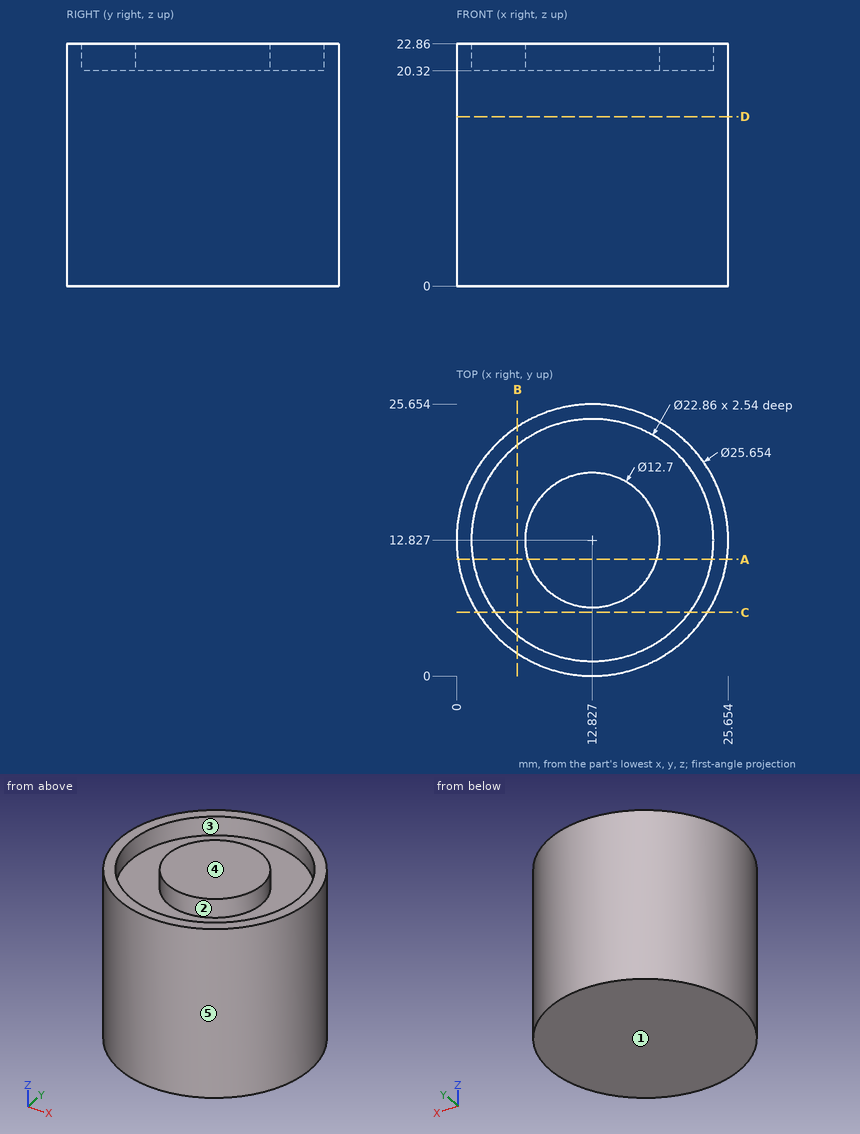
For this review, use the dimensioned drawing (mm, ordinates from the lowest corner) and the shaded views. A direction names the side the tool comes from. Coordinates: 2 decimals unless noted, no trailing zeros. Order: outer loops, then holes, each group sorted by start corner. A loop starts at its lowest first (then second) coordinate and runs counter-clockwise, first axis right, second up. Notation, with made-up numbers: M 39.25,56 L 96.25,56 A8 ccw 96.25,65 Z; hole C 85.5,78 d7. An arc over 180 degrees is marked long. Answer as a JSON object with one key per item and string values. Group by question number.
1) Add section C-C, the plane y = 6. Write out the cut boundary in (x, z).
2) Wall thickness on L1, parallel to Y at x = 17.75, z = 21.25; L2, parallel to Z at x = 10.75, y = 22.5; L3, parallel to Y at x = 19, z = 16: over which ranges is each line inside the solid? List them lowest first.
3) Add section D-D, the plane z = 16. Write out the cut boundary in (x, y), then the cut area to 3 significant figures.
4) Add section A-A, the plane y = 11. Write out the cut boundary in (x, z), then the cut area to 3 significant figures.
5) Tool access review of the marked faces 1 and 2: name each direction out of +Z, -Z, +X, -X, +Y, -Y from which nothing blocks a thin tool from reaching the whole face with its end or side.
6) Mouldability with a two-part tool opening along X and no side actions: class the marked faces 3, 4 and 5 as pulls with the +X half, pulls with the -X half, needs draft (parallel to the pull), parting line crosses it, or undercut.
7) Add section B-B, the plane x = 5.75. Write out the cut boundary in (y, z).
8) For pin 1 (1.5 mm diameter, centred on y = 8, z = 9.5, fed in from +X); pin 2 (4 mm diameter, centred on y = 4.5, z = 3, fed in from +X) (3 decimals); pin 3 (6 mm diameter, centred on x = 22, z = 19, fed in from -Y), all flat-tipped, find the tip position at first contact; note any pin that passes through.
Computed values:
{
 "1": {"outline": "M 1.97,0 L 23.69,0 L 23.69,22.86 L 21.99,22.86 L 21.99,20.32 L 3.66,20.32 L 3.66,22.86 L 1.97,22.86 Z"},
 "2": {"L1": "y = 0.98 to 2.51, 8.82 to 16.84, 23.14 to 24.67", "L2": "z = 0 to 20.32", "L3": "y = 1.58 to 24.07"},
 "3": {"outline": "C 12.83,12.83 d25.65", "area": "517 mm^2"},
 "4": {"outline": "M 0.13,0 L 25.52,0 L 25.52,22.86 L 24.11,22.86 L 24.11,20.32 L 18.91,20.32 L 18.91,22.86 L 6.75,22.86 L 6.75,20.32 L 1.54,20.32 L 1.54,22.86 L 0.13,22.86 Z", "area": "554 mm^2"},
 "5": {"face 1": "-Z, +X, -X, +Y, -Y", "face 2": "+Z"},
 "6": {"face 3": "undercut", "face 4": "needs draft", "face 5": "parting line crosses it"},
 "7": {"outline": "M 2.13,0 L 23.53,0 L 23.53,22.86 L 21.8,22.86 L 21.8,20.32 L 3.85,20.32 L 3.85,22.86 L 2.13,22.86 Z"},
 "8": {"pin 1": "stops at x = 24.99", "pin 2": "stops at x = 23.985", "pin 3": "stops at y = 1.58"}
}
